from build123d import *

# Parameters (mm, degrees)
SKETCH1_W           = 76.2
SKETCH1_H           = 76.2
SKETCH1_R           = 2.54
BOSS_EXTRUDE1_DEPTH = 2.54
FILLET1_R           = 7.62
FILLET2_R           = 7.62
FILLET3_R           = 7.62
FILLET4_R           = 7.62
CAVITY1_OUTLINE_R   = 2.413
CAVITY1_DEPTH       = 2.54


# Read off the part's stored shape, not the designer's step: Cavity1
with BuildPart() as part:
    # Sketch1 → Boss-Extrude1 (new body)
    with BuildSketch(Plane.XY):
        Rectangle(SKETCH1_W, SKETCH1_H)
        with Locations((-18.288, 25.4)):
            Circle(SKETCH1_R, mode=Mode.SUBTRACT)
        with Locations((18.288, 25.4)):
            Circle(SKETCH1_R, mode=Mode.SUBTRACT)
    extrude(amount=BOSS_EXTRUDE1_DEPTH)

    # Fillet1
    fillet1_edges = [part.edges().sort_by_distance(p)[0] for p in [
        (38.1, 38.1, 1.27),
    ]]
    fillet(fillet1_edges, radius=FILLET1_R)

    # Fillet2
    fillet2_edges = [part.edges().sort_by_distance(p)[0] for p in [
        (38.1, -38.1, 1.27),
    ]]
    fillet(fillet2_edges, radius=FILLET2_R)

    # Fillet3
    fillet3_edges = [part.edges().sort_by_distance(p)[0] for p in [
        (-38.1, -38.1, 1.27),
    ]]
    fillet(fillet3_edges, radius=FILLET3_R)

    # Fillet4
    fillet4_edges = [part.edges().sort_by_distance(p)[0] for p in [
        (-38.1, 38.1, 1.27),
    ]]
    fillet(fillet4_edges, radius=FILLET4_R)

    # Cavity1 outline → Cavity1 (cut)
    with BuildSketch(Plane.XY):
        with Locations((18.877459074, -25.789271924)):
            Circle(CAVITY1_OUTLINE_R)
        with Locations((-19.220954695, -25.105760078)):
            Circle(CAVITY1_OUTLINE_R)
    extrude(amount=CAVITY1_DEPTH, mode=Mode.SUBTRACT)


solid = part.part
Geometry: final body of the model. Coordinates: model frame, mm. Give positions to 0.01 mm unless a question says otherwise; leave off trailing zeros. Loops run counter-clockwise (first coordinate to the right, second up) from the corner with the lowest first, then second, coordinate; pieces in that order, holes last. Notation, with made-up numbers: M 55,-14 L 59,-14 A12 ccw 59,1 Z; hole C 21,2.5 d11. An arc over 180 degrees is marked long. Put each result on its own line as item: value. Start each with the question number.
1) Cut plane B-B (z = 1.45). Output: boundary loops of the cut face in (x, y), then the cut area to 3 significant figures.
2) Ray query, line 1 along X through (y, z) = (24, 0.95); line 2 along X through (y, z) = (26.5, 1.65); line 3 along Y through (x, z) = (-20, 1.6). Return the intervals inside material, ascending.
3) Pull-direction query (Y, two-part tool) for faces 1 (the cylindrical face through (35.927, -35.809, 1.288)), 2 (the flat face through (0, 38.1, 1)), 3 (the cylindrical face through (19.99, -27.93, 1.25)), 4 (the flat face through (-38.1, 0, 1)); classes: pulls with the +Y half, pulls with the -Y half, needs draft (parallel to the pull), parting line crosses it, or undercut.
4) Cut plane A-A (y = 25.4). Output: boundary loops of the cut face in (x, z).
Verdict:
1. outline: M -38.1,-30.48 A7.62 ccw -30.48,-38.1 L 30.48,-38.1 A7.62 ccw 38.1,-30.48 L 38.1,30.48 A7.62 ccw 30.48,38.1 L -30.48,38.1 A7.62 ccw -38.1,30.48 Z; hole C -19.22,-25.11 d4.83; hole C -18.29,25.4 d5.08; hole C 18.29,25.4 d5.08; hole C 18.88,-25.79 d4.83
1. area: 5,680 mm2
2. line 1: -38.1 to -20.41, -16.17 to 16.17, 20.41 to 38.1
2. line 2: -38.1 to -20.58, -16 to 16, 20.58 to 38.1
2. line 3: -38.1 to -27.39, -22.82 to 23.52, 27.28 to 38.1
3. face 1: pulls with the -Y half
3. face 2: pulls with the +Y half
3. face 3: undercut
3. face 4: needs draft
4. outline: M -38.1,0 L -20.83,0 L -20.83,2.54 L -38.1,2.54 Z; M -15.75,0 L 15.75,0 L 15.75,2.54 L -15.75,2.54 Z; M 20.83,0 L 38.1,0 L 38.1,2.54 L 20.83,2.54 Z
